CAD build for the part. Positions are in the model's coordinates, mm. Face numbers are marked on the shaded views. A direction names the side the tool comes from. Round coordinates to 2 decimals unless told otherwise and drop trailing zeros. Write each loop counter-clockwise with the first axis right and the second up, starting at its lowest first coordinate (ties: lowest second). Pieces come first, ordered by that corner, then holes. Notation, with made-up numbers: (46.5, 64.25) -> (70.5, 64.25) arc R8 ccw to (70.5, 68.25) -> close; hole circle Ø6 at (-15, -9.75). An arc over 180 degrees is marked (long way). Answer in a Markdown table with one row per item. Add a question column.
```python
from build123d import *

# Parameters (mm, degrees)
SZKIC2_W                         = 30
SZKIC2_H                         = 15
SZKIC2_R                         = 1
DODANIE_WYCI_GNI_CIE1_DEPTH      = 2.5
DODANIE_WYCI_GNI_CIE2_DEPTH      = 4
DODANIE_WYCI_GNI_CIE2_DEPTH_BACK = 6.5
SZKIC4_W                         = 30
SZKIC4_H                         = 4
SFAZOWANIE1_SIZE                 = 3
SFAZOWANIE1_SIZE2                = 0.974759089


with BuildPart() as part:
    # Szkic2 → Dodanie-wyciągnięcie1 (new body)
    with BuildSketch(Plane(origin=(0, 0, 0), x_dir=(1, 0, 0), z_dir=(0, 1, 0))):
        Rectangle(SZKIC2_W, SZKIC2_H)
        with Locations(Location((0, 2.5, 0), (0, 0, 270))):
            Circle(SZKIC2_R, mode=Mode.SUBTRACT)
    dodanie_wyci_gni_cie1 = extrude(amount=DODANIE_WYCI_GNI_CIE1_DEPTH)

    # Szkic4 → Dodanie-wyciągnięcie2 (add, two sides: drawn at the far end of the back side and taken through both)
    with BuildSketch(Plane(origin=(0, 2.5, 0), x_dir=(1, 0, 0), z_dir=(0, 1, 0)).offset(-DODANIE_WYCI_GNI_CIE2_DEPTH_BACK)):
        with Locations((0, -5.5)):
            Rectangle(SZKIC4_W, SZKIC4_H)
    extrude(amount=DODANIE_WYCI_GNI_CIE2_DEPTH + DODANIE_WYCI_GNI_CIE2_DEPTH_BACK)

    # Lustro3: Dodanie-wyciągnięcie1 across plane
    add(dodanie_wyci_gni_cie1.mirror(Plane.ZX.offset(4.5)))

    # Sfazowanie1
    sfazowanie1_edges = [part.edges().sort_by_distance(p)[0] for p in [
        (0, -4, 7.5),
    ]]
    sfazowanie1_side = [part.faces().sort_by_distance(p)[0] for p in [
        (0, -4, 5.5),
    ]]
    chamfer(sfazowanie1_edges, length=SFAZOWANIE1_SIZE, length2=SFAZOWANIE1_SIZE2, reference=sfazowanie1_side[0])


solid = part.part
```
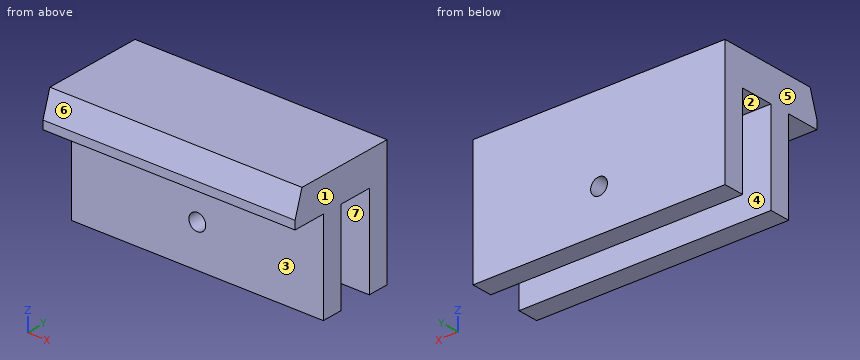
Item 1: Drill centre lines: probe 1 along Y at (x, z) = (-13.25, -6); probe 2 along X at (y, z) = (1.5, -2.5); probe 3 along Z at (x, y) = (5.75, -1.5). Where is each one in solid material? Low to high.
Item 2: Saw through at D-D on x = 7.5. Give the cut face in (y, z).
Item 3: Saw through at C-C on z = -2.5. Give the cut face in (x, y).
Item 4: Saw through at A-A on x = 0. Give the cut face in (y, z), then the cut area to 3 significant figures.
Item 5: Tool access for the marked faces 1, 2 and 3: list every direction of +Z, -Z, +X, -X, +Y, -Y with a clear straight run to the whole face (end or side of a thin tool).
Item 6: Pin check, flat tips, straight feed: pin 1 (2.5 mm diameter, centred on x = 0, z = -2.5, fed in from -Y); pin 2 (1.5 mm diameter, centred on y = -1.5, z = -2, fed in from -X); pin 3 (3 mm diameter, centred on x = -1.5, y = -2, fed in from -Z). Stop position of each tip, or through.
Item 7: Two-plate mould, pull along Y, no slides. Class the marked faces 4, 5, 6 and 7: +Y half, -Y half, draft (parallel to the pull), parting line (faces both ways), or undercut.
Item 8: Saw through at B-B on z = 2. Give the cut face in (x, y), then the cut area to 3 significant figures.
Recorded:
| question | item | result |
|---|---|---|
| 1 | probe 1 | 0 to 2.5, 6.5 to 9 |
| 1 | probe 2 | -15 to -1, 1 to 15 |
| 1 | probe 3 | 3.5 to 7.5 |
| 2 | outline | (-4, 3.5) -> (0, 3.5) -> (0, -7.5) -> (2.5, -7.5) -> (2.5, 3.5) -> (6.5, 3.5) -> (6.5, -7.5) -> (9, -7.5) -> (9, 7.5) -> (-3.03, 7.5) -> (-4, 4.5) -> close |
| 3 | outline | (-15, 0) -> (-1, 0) -> (-1, 2.5) -> (-15, 2.5) -> close; (-15, 6.5) -> (-1, 6.5) -> (-1, 9) -> (-15, 9) -> close; (1, 0) -> (15, 0) -> (15, 2.5) -> (1, 2.5) -> close; (1, 6.5) -> (15, 6.5) -> (15, 9) -> (1, 9) -> close |
| 4 | outline | (-4, 3.5) -> (0, 3.5) -> (0, -1.5) -> (2.5, -1.5) -> (2.5, 3.5) -> (6.5, 3.5) -> (6.5, -1.5) -> (9, -1.5) -> (9, 7.5) -> (-3.03, 7.5) -> (-4, 4.5) -> close; (0, -7.5) -> (2.5, -7.5) -> (2.5, -3.5) -> (0, -3.5) -> close; (6.5, -7.5) -> (9, -7.5) -> (9, -3.5) -> (6.5, -3.5) -> close |
| 4 | area | 95.5 mm2 |
| 5 | face 1 | +Z, -Z, +X, +Y, -Y |
| 5 | face 2 | -Z, +X, -X |
| 5 | face 3 | -Z, +X, -X, -Y |
| 6 | pin 1 | y = 0 |
| 6 | pin 2 | through |
| 6 | pin 3 | z = 3.5 |
| 7 | face 4 | undercut |
| 7 | face 5 | draft |
| 7 | face 6 | -Y half |
| 7 | face 7 | undercut |
| 8 | outline | (-15, 0) -> (15, 0) -> (15, 2.5) -> (-15, 2.5) -> close; (-15, 6.5) -> (15, 6.5) -> (15, 9) -> (-15, 9) -> close |
| 8 | area | 150 mm2 |
